Read the model definition and answer for the solid it produces. Units are mm, in the model's axes. Give positions to 0.01 mm unless a question says otherwise; leave off trailing zeros. Order: outer loops, then holes, each group sorted by start corner. A loop starts at its lowest first (then second) coordinate and runs counter-clockwise, first axis right, second up. Notation, with made-up numbers: M 29.25,-29 L 54.25,-29 A32 ccw 54.25,2 Z; hole C -8,-29.75 d11. An arc over 180 degrees is marked long. One line per item, written item: value.
from build123d import *

# Parameters (mm, degrees)
SKETCH2_W            = 130
SKETCH2_H            = 90
BOSS_EXTRUDE1_DEPTH  = 3
SKETCH3_R            = 1.5
CUT_EXTRUDE1_DEPTH   = 4
LPATTERN1_COUNT      = 2
LPATTERN1_PITCH      = 78
LPATTERN1_COUNT_DIR2 = 2
LPATTERN1_PITCH_DIR2 = 118


with BuildPart() as part:
    # Sketch2 → Boss-Extrude1 (new body)
    with BuildSketch(Plane(origin=(0, 0, 0), x_dir=(1, 0, 0), z_dir=(0, 1, 0))):
        Rectangle(SKETCH2_W, SKETCH2_H)
    extrude(amount=BOSS_EXTRUDE1_DEPTH)

    # Sketch3 → Cut-Extrude1 (cut, through all)
    with BuildSketch(Plane(origin=(0, 3, 0), x_dir=(1, 0, 0), z_dir=(0, 1, 0))):
        with Locations((59, -39)):
            Circle(SKETCH3_R)
    cut_extrude1 = extrude(amount=-CUT_EXTRUDE1_DEPTH, mode=Mode.SUBTRACT)

    # LPattern1: Cut-Extrude1 2 × 2
    with Locations(*[(-j * LPATTERN1_PITCH_DIR2, 0, -i * LPATTERN1_PITCH) for i in range(LPATTERN1_COUNT) for j in range(LPATTERN1_COUNT_DIR2) if (i, j) != (0, 0)]):
        add(cut_extrude1, mode=Mode.SUBTRACT)


solid = part.part
1) This flat-tipped pin is pushed along its axis until it touches: pin 1 Ø2.5 at (x, z) = (-59, -39) entering from -Y. Where does it stop, or does it pass through?
Reported:
pin 1: passes through
2) Determine the mould class of faces 1 (the face through (-57.614, 1.521, -38.425)), 2 (the face through (-65, 1, 1)), 3 (the face through (-1, 0, -1)), 4 (the face through (65, 1, 1)) for opening direction X: +X half, -X half, draft (parallel to the pull), parting line (faces both ways), or undercut.
Reported:
face 1: undercut
face 2: -X half
face 3: draft
face 4: +X half
3) Find section B-B, the plane z = -39. Write down the section's boundary in (x, y).
Reported:
outline: M -65,0 L -60.5,0 L -60.5,3 L -65,3 Z; M -57.5,0 L 57.5,0 L 57.5,3 L -57.5,3 Z; M 60.5,0 L 65,0 L 65,3 L 60.5,3 Z
4) Consider probe 1 along Z at (x, y) = (59, 1.8); probe 2 along X at (y, z) = (2.4, -39); probe 3 along Z at (x, y) = (60, 0.6). Determine where each line is inside the solid, lowest interval first.
Reported:
probe 1: z = -45 to -40.5, -37.5 to 37.5, 40.5 to 45
probe 2: x = -65 to -60.5, -57.5 to 57.5, 60.5 to 65
probe 3: z = -45 to -40.12, -37.88 to 37.88, 40.12 to 45
5) Find section A-A, the plane x = -59. Write down the section's boundary in (y, z).
Reported:
outline: M 0,-45 L 3,-45 L 3,-40.5 L 0,-40.5 Z; M 0,-37.5 L 3,-37.5 L 3,37.5 L 0,37.5 Z; M 0,40.5 L 3,40.5 L 3,45 L 0,45 Z
